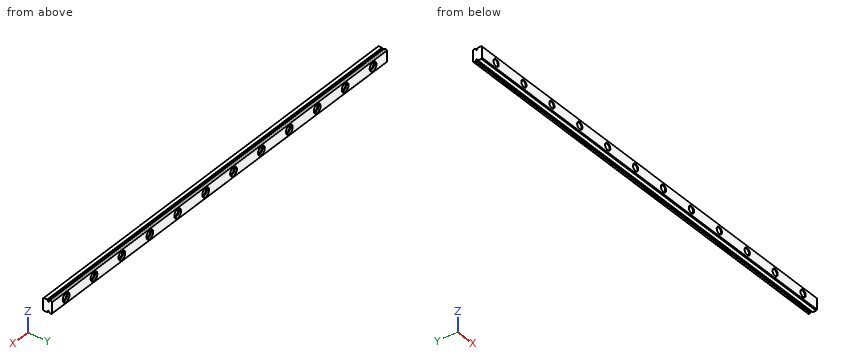
from build123d import *

# Parameters (mm, degrees)
EXTRUDE1_DEPTH  = 180
LPATTERN1_COUNT = 11
LPATTERN1_PITCH = 15


with BuildPart() as part:
    # Sketch1 → Extrude1 (new body)
    with BuildSketch(Plane(origin=(0, 0, 0), x_dir=(0, 0, -1), z_dir=(1, 0, 0))):
        with BuildLine():
            Line((-2.5, 0.3), (-2.2, 0))
            Line((-2.2, 0), (2.2, 0))
            Line((2.2, 0), (2.5, 0.3))
            Line((2.5, 0.3), (2.5, 1.723030399))
            ThreePointArc((2.5, 1.723030399), (2.315825857, 1.828075757), (2.191742431, 2))
            Line((2.191742431, 2), (1.85, 2))
            ThreePointArc((1.85, 2), (1.779289322, 2.029289322), (1.75, 2.1))
            Line((1.75, 2.1), (1.75, 2.3))
            ThreePointArc((1.75, 2.3), (1.779289322, 2.370710678), (1.85, 2.4))
            Line((1.85, 2.4), (2.191742431, 2.4))
            ThreePointArc((2.191742431, 2.4), (2.315825857, 2.571924243), (2.5, 2.676969601))
            Line((2.5, 2.676969601), (2.5, 3.3))
            ThreePointArc((2.5, 3.3), (2.393651515, 3.532738637), (2.2, 3.7))
            Line((2.2, 3.7), (-2.2, 3.7))
            ThreePointArc((-2.2, 3.7), (-2.393651515, 3.532738637), (-2.5, 3.3))
            Line((-2.5, 3.3), (-2.5, 2.676969601))
            ThreePointArc((-2.5, 2.676969601), (-2.315825857, 2.571924243), (-2.191742431, 2.4))
            Line((-2.191742431, 2.4), (-1.85, 2.4))
            ThreePointArc((-1.85, 2.4), (-1.779289322, 2.370710678), (-1.75, 2.3))
            Line((-1.75, 2.3), (-1.75, 2.1))
            ThreePointArc((-1.75, 2.1), (-1.779289322, 2.029289322), (-1.85, 2))
            Line((-1.85, 2), (-2.191742431, 2))
            ThreePointArc((-2.191742431, 2), (-2.315825857, 1.828075757), (-2.5, 1.723030399))
            Line((-2.5, 1.723030399), (-2.5, 0.3))
        make_face()
    extrude(amount=EXTRUDE1_DEPTH)

    # Sketch2 → Cut-Revolve1 (revolve, cut)
    with BuildSketch(Plane(origin=(0, 0, 0), x_dir=(-1, 0, 0), z_dir=(0, 0, -1)), mode=Mode.PRIVATE) as cut_revolve1_sk:
        Polygon((-7.5, 3.7), (-5.7, 3.7), (-5.7, 2.9), (-6.3, 2.9), (-6.3, 0.2), (-6.1, 0), (-7.5, 0), align=None)
    revolve(cut_revolve1_sk.sketch.rotate(Axis((7.5, 0, 0), (0, 1, 0)), 90), axis=Axis((7.5, 0, 0), (0, 1, 0)), mode=Mode.SUBTRACT)

    # Sketch3 → Cut-Revolve2 (revolve, cut)
    with BuildSketch(Plane(origin=(45, 0, 0), x_dir=(-1, 0, 0), z_dir=(0, 0, -1)), mode=Mode.PRIVATE) as cut_revolve2_sk:
        Polygon((-127.5, 3.7), (-125.7, 3.7), (-125.7, 2.9), (-126.3, 2.9), (-126.3, 0.2), (-126.1, 0), (-127.5, 0), align=None)
    cut_revolve2 = revolve(cut_revolve2_sk.sketch.rotate(Axis((172.5, 0, 0), (0, 1, 0)), 90), axis=Axis((172.5, 0, 0), (0, 1, 0)), mode=Mode.SUBTRACT)

    # LPattern1: Cut-Revolve2 ×11
    with Locations(*[(-i * LPATTERN1_PITCH, 0, 0) for i in range(1, LPATTERN1_COUNT)]):
        add(cut_revolve2, mode=Mode.SUBTRACT)


solid = part.part
Could you check a few things on this model? Use its own coordinates, in mm. Coordinates: 2 decimals unless noted, no trailing zeros. Order: outer loops, then holes, each group sorted by start corner. A loop starts at its lowest first (then second) coordinate and runs counter-clockwise, first axis right, second up.
Q1. Will this pin go through, and if not, where does the flat tip stop? pin 1 (3 mm diameter, centred on x = 37.5, z = 0, fed in from +Y).
Q2. Suppose I cut it at B-B on z = 0. Give the number of separate pieces and of enclosed holes in the cut face, and give its area (3 significant figures).
Q3. Please list where these lines run through material, in increasing order: L1, parallel to Y at x = 57.5, z = -2; L2, parallel to Z at x = 97, y = 1.35; L3, parallel to Z at x = 38.5, y = 2.65.
Q4. Suppose I cut it at A-A on x = 149. Please give me the cut outline in (y, z).
Answer:
1. pin 1: stops at y = 2.9
2. separate pieces: 13
2. enclosed holes: 0
2. area: 547 mm2
3. L1: y = 0 to 2, 2.4 to 3.7
3. L2: z = -2.5 to -1.09, 1.09 to 2.5
3. L3: z = -2.43 to -0.66, 0.66 to 2.43
4. outline: (0, -2.2) - (0.3, -2.5) - (1.72, -2.5) arc R0.5 cw to (2, -2.19) - (2, -1.85) arc R0.1 cw to (2.1, -1.75) - (2.3, -1.75) arc R0.1 cw to (2.4, -1.85) - (2.4, -2.19) arc R0.5 cw to (2.68, -2.5) - (3.3, -2.5) arc R0.6 ccw to (3.7, -2.2) - (3.7, 2.2) arc R0.6 ccw to (3.3, 2.5) - (2.68, 2.5) arc R0.5 cw to (2.4, 2.19) - (2.4, 1.85) arc R0.1 cw to (2.3, 1.75) - (2.1, 1.75) arc R0.1 cw to (2, 1.85) - (2, 2.19) arc R0.5 cw to (1.72, 2.5) - (0.3, 2.5) - (0, 2.2) - close
